Read the model definition and answer for the solid it produces. Units are mm, in the model's axes. Face numbers are marked on the shaded views. A direction names the side the tool comes from. Give positions to 0.01 mm unless a question says otherwise; leave off trailing zeros. Order: outer loops, then holes, each group sorted by start corner. A loop starts at its lowest first (then second) coordinate and runs counter-clockwise, first axis right, second up.
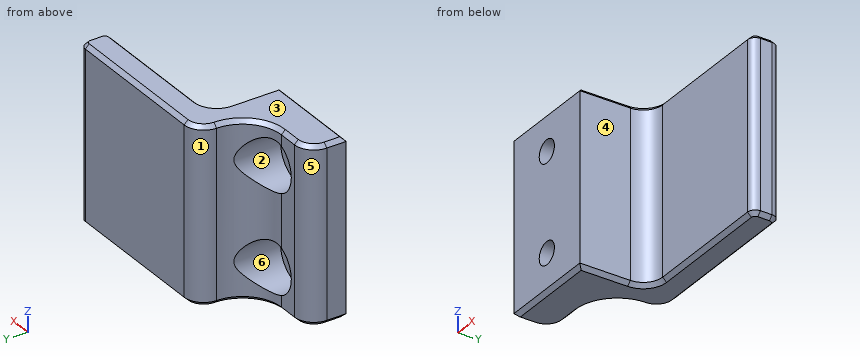
```python
from build123d import *

# Parameters (mm, degrees)
BOSS_EXTRUDE1_DEPTH = 22.5
SKETCH3_R           = 2.921
CUT_EXTRUDE1_DEPTH  = 51.204979833
SKETCH3_4_R         = 6.5
SKETCH3_4_R_2       = 2.921
CUT_EXTRUDE2_DEPTH  = 6
FILLET1_R           = 10
FILLET2_R           = 5
FILLET4_R           = 2
CHAMFER1_SIZE       = 1


# Some blends are built 0.0001 mm under size
with BuildPart() as part:
    # Sketch1 → Boss-Extrude1 (new, symmetric)
    with BuildSketch(Plane.XY):
        Polygon((-22.7, -12.5), (2.7, -12.5), (2.7, 5.5), (42.3, 5.5), (42.3, 12.5), (-2.7, 12.5), (-2.7, -2.5), (-22.7, -2.5), align=None)
    extrude(amount=BOSS_EXTRUDE1_DEPTH, both=True)

    # Sketch3 → Cut-Extrude1 (cut, through all)
    with BuildSketch(Plane(origin=(0, -2.5, 0), x_dir=(1, 0, 0), z_dir=(0, 1, 0))):
        with Locations(Location((-10, -12.7, 0), (0, 0, 180))):
            Circle(SKETCH3_R)
    cut_extrude1 = extrude(amount=-CUT_EXTRUDE1_DEPTH, mode=Mode.SUBTRACT)

    # Sketch3<4> → Cut-Extrude2 (cut)
    with BuildSketch(Plane(origin=(0, -2.5, 0), x_dir=(1, 0, 0), z_dir=(0, 1, 0))):
        with Locations(Location((-10, -12.7, 0), (0, 0, 180))):
            Circle(SKETCH3_4_R)
        with Locations(Location((-10, -12.7, 0), (0, 0, 180))):
            Circle(SKETCH3_4_R_2, mode=Mode.SUBTRACT)
    cut_extrude2 = extrude(amount=-CUT_EXTRUDE2_DEPTH, mode=Mode.SUBTRACT)

    # Mirror1: Cut-Extrude1, Cut-Extrude2 across plane
    add(cut_extrude1.mirror(Plane.XY), mode=Mode.SUBTRACT)
    add(cut_extrude2.mirror(Plane.XY), mode=Mode.SUBTRACT)

    # Fillet1
    # the kernel refuses this fillet: 10 mm, written as the material it adds along each edge
    with BuildSketch(Plane(origin=(-2.7, -2.5, 22.5), x_dir=(0, 1, 0), z_dir=(0, 0, -1))) as fillet1_piece_1_section:
        with BuildLine():
            CenterArc((FILLET1_R, -FILLET1_R), FILLET1_R, 90, 90)
            Line((0, -FILLET1_R), (0, 0))
            Line((0, 0), (FILLET1_R, 0))
        make_face()
    fillet1_piece_1 = extrude(amount=45, mode=Mode.PRIVATE)
    fillet1_piece_1 = fillet1_piece_1 - Plane(origin=(-10, 0.155378063, -12.7), x_dir=(-1, 0, 0), z_dir=(0, 1, 0)) * Cylinder(6.5, 130, mode=Mode.PRIVATE)
    fillet1_piece_1 = fillet1_piece_1 - Plane(origin=(-10, 0.155378063, 12.7), x_dir=(-1, 0, 0), z_dir=(0, 1, 0)) * Cylinder(6.5, 130, mode=Mode.PRIVATE)
    add(fillet1_piece_1)

    # Fillet2
    fillet2_edges = [part.edges().sort_by_distance(p)[0] for p in [
        (2.7, 5.5, 0),
        (-22.7, -2.5, 0),
        (-2.7, 12.5, 0),
    ]]
    fillet(fillet2_edges, radius=FILLET2_R - 0.0001)  # a hair under: the kernel refuses the full size

    # Fillet4
    fillet4_edges = [part.edges().sort_by_distance(p)[0] for p in [
        (42.3, 12.5, 0),
        (42.3, 5.5, 0),
    ]]
    fillet(fillet4_edges, radius=FILLET4_R)

    # Chamfer1
    chamfer1_edges = [part.edges().sort_by_distance(p)[0] for p in [
        (2.7, -5.99995, -22.5),
        (-10, -12.5, -22.5),
        (2.7, -5.99995, 22.5),
        (-15.20005, -2.5, -22.5),
        (-15.20005, -2.5, 22.5),
        (-5.628932188, 0.428932188, -22.5),
        (-5.628932188, 0.428932188, 22.5),
        (-22.7, -9.99995, -22.5),
        (-22.7, -9.99995, 22.5),
        (23.99995, 5.5, -22.5),
        (-1.235563195, 11.035563195, -22.5),
        (-21.235563195, -3.964436805, -22.5),
        (23.99995, 5.5, 22.5),
        (-1.235563195, 11.035563195, 22.5),
        (-21.235563195, -3.964436805, 22.5),
        (4.164436805, 4.035563195, -22.5),
        (4.164436805, 4.035563195, 22.5),
        (21.29995, 12.5, -22.5),
        (21.29995, 12.5, 22.5),
        (42.3, 9, -22.5),
        (41.714213562, 6.085786438, -22.5),
        (41.714213562, 11.914213562, -22.5),
        (42.3, 9, 22.5),
        (41.714213562, 6.085786438, 22.5),
        (41.714213562, 11.914213562, 22.5),
        (-10, -12.5, 22.5),
    ]]
    chamfer(chamfer1_edges, length=CHAMFER1_SIZE)


solid = part.part
```
1) Given pin 1 (4 mm diameter, centred on y = 3, z = 14, fed in from +X); pin 2 (1 mm diameter, centred on y = 5, z = -16, fed in from -X); pin 3 (5.5 mm diameter, centred on x = -10, z = 12.7, fed in from +Y); pin 4 (12 mm diameter, centred on x = 3, y = 0, fed in from -Z), each flat-ended and moving along its own axis, determine where each tip first touches the part or whether it passes through.
Final values:
pin 1: stops at x = 5.52
pin 2: stops at x = -3.16
pin 3: passes through
pin 4: stops at z = -22.5
2) The part is cut by section B-B on x = 15. Determine the outline of the cut face in (y, z).
Final values:
outline: (5.5, -21.5) - (6.5, -22.5) - (11.5, -22.5) - (12.5, -21.5) - (12.5, 21.5) - (11.5, 22.5) - (6.5, 22.5) - (5.5, 21.5) - close
3) A tool of negligible diameter and unlimited length cuts with its end or side. For the marked faces 4, 5 and 6, from which of +Z, -Z, +X, -X, +Y, -Y can it reach the whole face along a straight path? Write none if from no direction.
Final values:
face 4: +Z, -Z, +X, -Y
face 5: +Z, -Z, -X, +Y
face 6: +Y
4) Consider L1, parallel to Z at x = -10, y = -11.5; L2, parallel to Z at x = -10, y = -5.75; L3, parallel to Y at x = 31, z = 12. Determine where each line is inside the solid, lowest interval first.
Final values:
L1: z = -22.5 to -15.62, -9.78 to 9.78, 15.62 to 22.5
L2: z = -22.5 to -19.2, -6.2 to 6.2, 19.2 to 22.5
L3: y = 5.5 to 12.5
5) For a pull along X with two mould halves and no side action, classify the marked faces 1, 2 and 3 as released by +X, released by -X, zero draft, split by the parting line, or undercut.
Final values:
face 1: released by -X
face 2: undercut
face 3: zero draft
6) The part is cut by section D-D on x = -10. Count the separate pieces of the cut face and the enclosed holes in it, and give its area (3 significant figures).
Final values:
separate pieces: 3
enclosed holes: 0
area: 252 mm2
